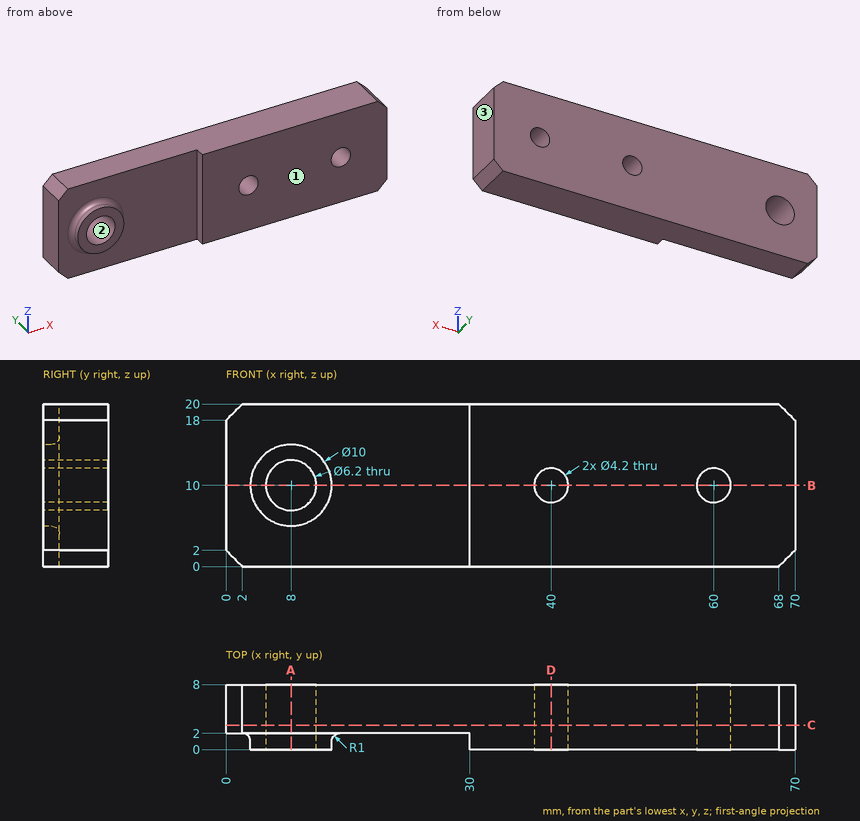
Print and shaded views of the part. All mm, measured from the part's lowest x, y and z. Round coordinates to 2 decimals unless told otherwise and drop trailing zeros. Write each loop counter-clockwise with the first axis right and the second up, starting at its lowest first coordinate (ties: lowest second). Pieces come first, ordered by that corner, then holes. Notation, with made-up numbers: (-34, 44) -> (-15, 44) arc R25 cw to (-15, 62) -> close; hole circle Ø9 at (-4.75, 9.5). An arc over 180 degrees is marked (long way). Answer in a Markdown table with one row per item. Add a question column.
Item 1: Saw through at D-D, the plane x = 40. Write the cut outline in (y, z), then the cut area to 3 significant figures.
Item 2: Drop flat-ended pins along their axis: pin 1 Ø3.5 at (x, z) = (40, 10) entering from +Y; pin 2 Ø1 at (x, z) = (48.5, 10.5) entering from -Y; pin 3 Ø1 at (x, z) = (19.5, 9) entering from -Y; pin 4 Ø1.6 at (y, z) = (1, 8.5) entering from -X. Give the stop position or say it passes through.
Item 3: Drill centre lines: line 1 (Z direction, x = 60, y = 5.5); line 2 (X direction, y = 7, z = 11); line 3 (X direction, y = 7.75, z = 11.75). Where is each one in solid material? Low to high. Write a range as from..to.
Item 4: Saw through at A-A, the plane x = 8. Write the cut outline in (y, z), then the cut area to 3 significant figures.
Item 5: Mould opens along X. For the marked faces 1, 2 and 3 say: pulls with the +X half, pulls with the -X half, needs draft (parallel to the pull), parting line crosses it, or undercut.
Item 6: Saw through at C-C, the plane y = 3. Write the cut outline in (x, z).
Item 7: Saw through at B-B, the plane z = 10. Write the cut outline in (x, y), then the cut area to 3 significant figures.
Findings below:
| question | item | result |
|---|---|---|
| 1 | outline | (0, 0) -> (8, 0) -> (8, 7.9) -> (0, 7.9) -> close; (0, 12.1) -> (8, 12.1) -> (8, 20) -> (0, 20) -> close |
| 1 | area | 126 mm^2 |
| 2 | pin 1 | passes through |
| 2 | pin 2 | stops at y = 0 |
| 2 | pin 3 | stops at y = 2 |
| 2 | pin 4 | stops at x = 2.79 |
| 3 | line 1 | z = 0..7.9, 12.1..20 |
| 3 | line 2 | x = 0..5.07, 10.93..38.15, 41.85..58.15, 61.85..70 |
| 3 | line 3 | x = 0..5.44, 10.56..38.84, 41.16..58.84, 61.16..70 |
| 4 | outline | (0, 5) -> (1, 5) arc R1 cw to (2, 4) -> (2, 0) -> (8, 0) -> (8, 6.9) -> (0, 6.9) -> close; (0, 13.1) -> (8, 13.1) -> (8, 20) -> (2, 20) -> (2, 16) arc R1 cw to (1, 15) -> (0, 15) -> close |
| 4 | area | 90.8 mm^2 |
| 5 | face 1 | needs draft |
| 5 | face 2 | undercut |
| 5 | face 3 | pulls with the +X half |
| 6 | outline | (0, 2) -> (2, 0) -> (68, 0) -> (70, 2) -> (70, 18) -> (68, 20) -> (2, 20) -> (0, 18) -> close; hole circle Ø6.2 at (8, 10); hole circle Ø4.2 at (40, 10); hole circle Ø4.2 at (60, 10) |
| 7 | outline | (0, 2) -> (2, 2) arc R1 cw to (3, 1) -> (3, 0) -> (4.9, 0) -> (4.9, 8) -> (0, 8) -> close; (11.1, 0) -> (13, 0) -> (13, 1) arc R1 cw to (14, 2) -> (30, 2) -> (30, 0) -> (37.9, 0) -> (37.9, 8) -> (11.1, 8) -> close; (42.1, 0) -> (57.9, 0) -> (57.9, 8) -> (42.1, 8) -> close; (62.1, 0) -> (70, 0) -> (70, 8) -> (62.1, 8) -> close |
| 7 | area | 404 mm^2 |
